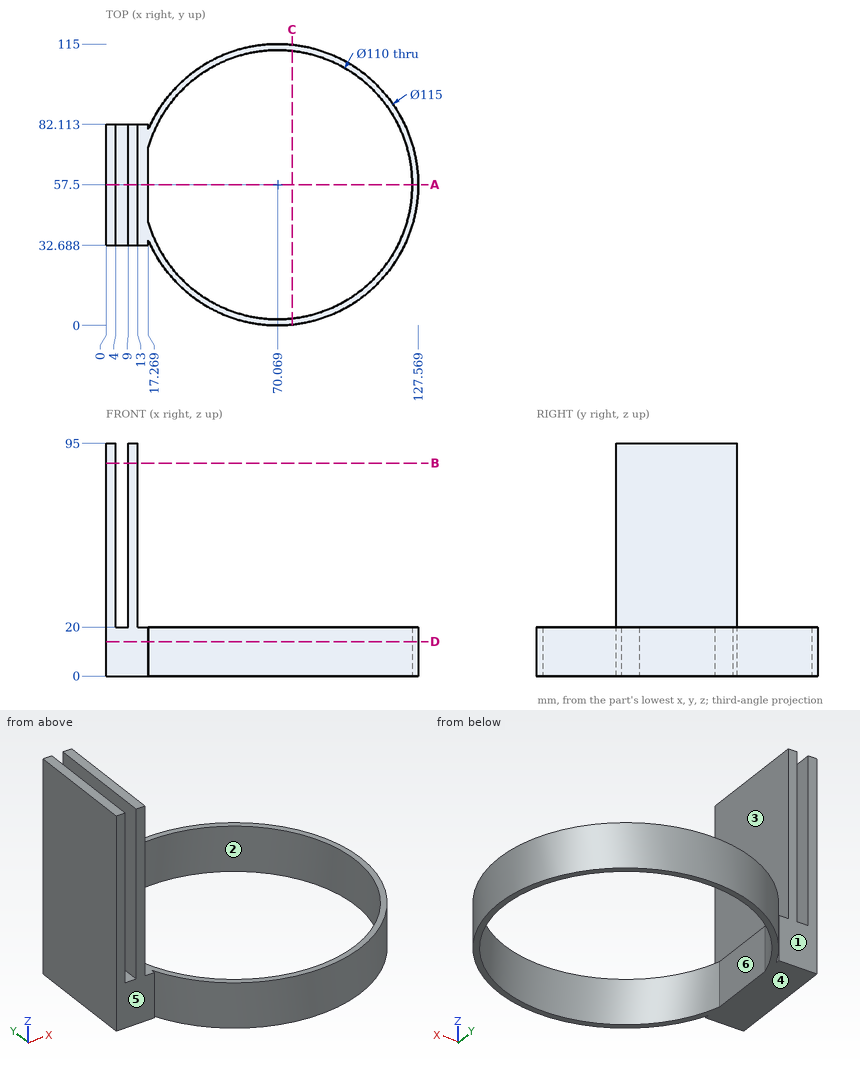
The drawing under review shows one solid part. Ordinate dimensions are in mm from its lowest x, y, z. A direction names the side the tool comes from. Coordinates: 2 decimals unless noted, no trailing zeros. Loops run counter-clockwise (first coordinate to the right, second up) from the corner with the lowest first, then second, coordinate; pieces in that order, holes last.
Item 1: Add section A-A (y = 57.5). Write out the cut boundary in (x, z).
Completed:
outline: (0, 0) - (17.27, 0) - (17.27, 20) - (13, 20) - (13, 95) - (9, 95) - (9, 20) - (4, 20) - (4, 95) - (0, 95) - close; (125.07, 0) - (127.57, 0) - (127.57, 20) - (125.07, 20) - close
Item 2: Add section D-D (z = 14). Write out the cut boundary in (x, y).
Completed:
outline: (0, 32.69) - (17.27, 32.69) - (17.27, 34.73) arc R57.5 ccw (long way) to (17.27, 80.27) - (17.27, 82.11) - (0, 82.11) - close; hole (17.27, 42.1) arc R55 ccw (long way) to (17.27, 72.9) - close
Item 3: Add section B-B (z = 87). Write out the cut boundary in (x, y).
Completed:
outline: (0, 32.69) - (4, 32.69) - (4, 82.11) - (0, 82.11) - close; (9, 32.69) - (13, 32.69) - (13, 82.11) - (9, 82.11) - close
Item 4: Clearance check with flat-ended pins moving along their axes: pin 1 (15 mm diameter, centred on y = 65.5, z = 58.5, fed in from +X); pin 2 (1 mm diameter, centred on y = 34, z = 10, fed in from +X); pin 3 (0.9 mm diameter, centred on y = 81.5, z = 9, fed in from +X) (1 decimal). State where each tip first meets the part, or that it passes through.
Completed:
pin 1: stops at x = 13
pin 2: stops at x = 122.77
pin 3: stops at x = 122.5
Item 5: Add section C-C (x = 76). Write out the cut boundary in (y, z).
Completed:
outline: (0.31, 0) - (2.82, 0) - (2.82, 20) - (0.31, 20) - close; (112.18, 0) - (114.69, 0) - (114.69, 20) - (112.18, 20) - close
Item 6: Wall thickness on L1, parallel to X at y = 82, z = 67.5; L2, parallel to X at y = 57, z = 15; L3, parallel to Z at x = 42.5, y = 105.5: over which ranges is each line inside the solid? List them lowest first.
Completed:
L1: x = 0 to 4, 9 to 13
L2: x = 0 to 17.27, 125.07 to 127.57
L3: z = 0 to 20
Item 7: Draft analysis for pull direction Y (two halves, no side actions). For the marked faces 4, 5 and 6, state which applies: pulls with the +Y half, pulls with the -Y half, needs draft (parallel to the pull), parting line crosses it, or undercut.
Completed:
face 4: needs draft
face 5: pulls with the -Y half
face 6: undercut
Item 8: For the marked faces 1, 2 and 3, list the 3-axis set-ups (+Z, -Z, +X, -X, +Y, -Y) from which the entire face can be reached by the end or side of a thin tool; tool diameter is ignored.
Completed:
face 1: +Z, -Z, -X, +Y
face 2: +Z, -Z
face 3: +Z, +X, +Y, -Y
